For this review, take the finished solid that the model builds, in its own axes (mm). Face numbers are marked on the shaded views. A direction names the side the tool comes from. Coordinates: 2 decimals unless noted, no trailing zeros. Write each loop counter-clockwise with the first axis right and the second up, starting at its lowest first coordinate (ties: lowest second). Pieces come first, ordered by that corner, then holes.
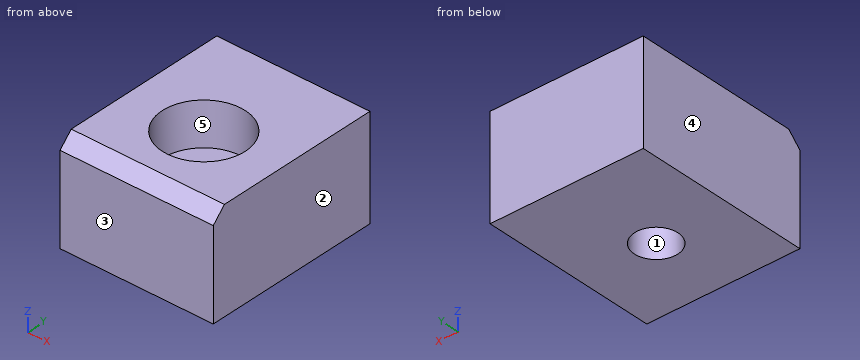
```python
from build123d import *

# Parameters (mm, degrees)
F0_W           = 12
F0_H           = 14
F1_DEPTH       = 8
F2_SIZE        = 1
F4_D           = 3.4
F4_DEPTH       = 10
F4_CBORE_D     = 6.5
F4_CBORE_DEPTH = 3.4


with BuildPart() as f1:
    # F0 (on Top) → F1 (new body)
    with BuildSketch(Plane.XY):
        Rectangle(F0_W, F0_H)
    extrude(amount=F1_DEPTH)

    # F2
    f2_edges = [f1.edges().sort_by_distance(p)[0] for p in [
        (0, -7, 8),
    ]]
    chamfer(f2_edges, length=F2_SIZE)

    # F4
    with Locations(Plane.XY.offset(8)):
        with Locations((0, -1)):
            CounterBoreHole(F4_D / 2, F4_CBORE_D / 2, F4_CBORE_DEPTH, depth=F4_DEPTH)


solid = f1.part
```
Q1. Tool access review of the marked faces 4 and 5: name each direction out of +Z, -Z, +X, -X, +Y, -Y from which nothing blocks a thin tool from reaching the whole face with its end or side.
Ans:
face 4: +Z, -Z, -X, +Y, -Y
face 5: +Z
Q2. Draft analysis for pull direction Y (two halves, no side actions). For the marked faces 1, 2 and 3, state which applies: +Y half, -Y half, draft (parallel to the pull), parting line (faces both ways), or undercut.
Ans:
face 1: undercut
face 2: draft
face 3: -Y half
Q3. Add section D-D (x = 2). State the section outline as (y, z) points, then the cut area to 3 significant figures.
Ans:
outline: (-7, 0) - (7, 0) - (7, 8) - (1.56, 8) - (1.56, 4.6) - (-3.56, 4.6) - (-3.56, 8) - (-6, 8) - (-7, 7) - close
area: 94.1 mm2
Q4. Add section C-C (z = 2). State the section outline as (x, y) points.
Ans:
outline: (-6, -7) - (6, -7) - (6, 7) - (-6, 7) - close; hole circle Ø3.4 at (0, -1)
Q5. Clearance check with a flat-ended pin moving along its axis: pin 1 Ø2.5 at (x, y) = (0, -1) entering from +Z. State where the tip first meets the part, or that it passes through.
Ans:
pin 1: passes through
Q6. For probe 1 along Y at (x, z) = (0, 1.1); probe 2 along Y at (x, z) = (0, 4.75); probe 3 along Z at (x, y) = (1, 1.25), list the stretches that pass through material, from the lowest coordinate up.
Ans:
probe 1: y = -7 to -2.7, 0.7 to 7
probe 2: y = -7 to -4.25, 2.25 to 7
probe 3: z = 0 to 4.6
Q7. Add section A-A (x = 0). State the section outline as (y, z) points, then the cut area to 3 significant figures.
Ans:
outline: (-7, 0) - (-2.7, 0) - (-2.7, 4.6) - (-4.25, 4.6) - (-4.25, 8) - (-6, 8) - (-7, 7) - close; (0.7, 0) - (7, 0) - (7, 8) - (2.25, 8) - (2.25, 4.6) - (0.7, 4.6) - close
area: 73.8 mm2
Q8. Add section B-B (y = -1). State the section outline as (x, z) points, then the cut area to 3 significant figures.
Ans:
outline: (-6, 0) - (-1.7, 0) - (-1.7, 4.6) - (-3.25, 4.6) - (-3.25, 8) - (-6, 8) - close; (1.7, 0) - (6, 0) - (6, 8) - (3.25, 8) - (3.25, 4.6) - (1.7, 4.6) - close
area: 58.3 mm2
